The model under review builds one solid part; all positions refer to its coordinate system, in mm. Round coordinates to 2 decimals unless told otherwise and drop trailing zeros. Write each loop counter-clockwise with the first axis right and the second up, starting at its lowest first coordinate (ties: lowest second). Pieces come first, ordered by that corner, then holes. Notation, with made-up numbers: (58.25, -38.5) - (112.25, -38.5) arc R26 cw to (112.25, -17.5) - close; hole circle Ø10 at (46.5, 16). An arc over 180 degrees is marked (long way). Use one line per item in the form item = value.
from build123d import *

# Parameters (mm, degrees)
BOSS_EXTRUDE1_DEPTH = 5


with BuildPart() as part:
    # Sketch1 → Boss-Extrude1 (new body)
    with BuildSketch(Plane(origin=(0, 0, 0), x_dir=(1, 0, 0), z_dir=(0, 1, 0))):
        with BuildLine():
            ThreePointArc((-7.859375, 1.493393655), (-5.656854249, 5.656854249), (-1.493393655, 7.859375))
            ThreePointArc((-1.493393655, 7.859375), (-1.109264959, 9.009718401), (0, 9.5))
            Line((0, 9.5), (0, 15))
            ThreePointArc((0, 15), (-15, 0), (0, -15))
            Line((0, -15), (0, -9.5))
            ThreePointArc((0, -9.5), (-1.109264959, -9.009718401), (-1.493393655, -7.859375))
            ThreePointArc((-1.493393655, -7.859375), (-5.656854249, -5.656854249), (-7.859375, -1.493393655))
            ThreePointArc((-7.859375, -1.493393655), (-9.5, 0), (-7.859375, 1.493393655))
        make_face()
        with BuildLine():
            ThreePointArc((1.5, 8), (1.498347504, 7.929609954), (1.493393655, 7.859375))
            ThreePointArc((1.493393655, 7.859375), (5.656854249, 5.656854249), (7.859375, 1.493393655))
            ThreePointArc((7.859375, 1.493393655), (9.009718401, 1.109264959), (9.5, 0))
            ThreePointArc((9.5, 0), (9.009718401, -1.109264959), (7.859375, -1.493393655))
            ThreePointArc((7.859375, -1.493393655), (5.656854249, -5.656854249), (1.493393655, -7.859375))
            ThreePointArc((1.493393655, -7.859375), (1.498347504, -7.929609954), (1.5, -8))
            ThreePointArc((1.5, -8), (1.060660172, -9.060660172), (0, -9.5))
            Line((0, -9.5), (0, -15))
            ThreePointArc((0, -15), (10.606601718, -10.606601718), (15, 0))
            ThreePointArc((15, 0), (10.606601718, 10.606601718), (0, 15))
            Line((0, 15), (0, 9.5))
            ThreePointArc((0, 9.5), (1.060660172, 9.060660172), (1.5, 8))
        make_face()
        with BuildLine():
            ThreePointArc((0, -5), (-5, 0), (0, 5))
            Line((0, 5), (0, 6.5))
            ThreePointArc((0, 6.5), (-1.009718401, 6.890735041), (-1.493393655, 7.859375))
            ThreePointArc((-1.493393655, 7.859375), (-5.656854249, 5.656854249), (-7.859375, 1.493393655))
            ThreePointArc((-7.859375, 1.493393655), (-6.890735041, 1.009718401), (-6.5, 0))
            ThreePointArc((-6.5, 0), (-6.890735041, -1.009718401), (-7.859375, -1.493393655))
            ThreePointArc((-7.859375, -1.493393655), (-5.656854249, -5.656854249), (-1.493393655, -7.859375))
            ThreePointArc((-1.493393655, -7.859375), (-1.009718401, -6.890735041), (0, -6.5))
            Line((0, -6.5), (0, -5))
        make_face()
        with BuildLine():
            Line((0, 6.5), (0, 5))
            ThreePointArc((0, 5), (3.535533906, 3.535533906), (5, 0))
            ThreePointArc((5, 0), (3.535533906, -3.535533906), (0, -5))
            Line((0, -5), (0, -6.5))
            ThreePointArc((0, -6.5), (1.009718401, -6.890735041), (1.493393655, -7.859375))
            ThreePointArc((1.493393655, -7.859375), (5.656854249, -5.656854249), (7.859375, -1.493393655))
            ThreePointArc((7.859375, -1.493393655), (6.5, 0), (7.859375, 1.493393655))
            ThreePointArc((7.859375, 1.493393655), (5.656854249, 5.656854249), (1.493393655, 7.859375))
            ThreePointArc((1.493393655, 7.859375), (1.009718401, 6.890735041), (0, 6.5))
        make_face()
        with BuildLine():
            Line((40, 15), (0, 15))
            ThreePointArc((0, 15), (10.606601718, 10.606601718), (15, 0))
            ThreePointArc((15, 0), (10.606601718, -10.606601718), (0, -15))
            Line((0, -15), (40, -15))
            Line((40, -15), (40, 15))
        make_face()
    extrude(amount=BOSS_EXTRUDE1_DEPTH)


solid = part.part
(1) Add section C-C on z = 3.5. Write out the cut boundary in (x, y).
Geometry results:
outline = (-14.59, 0) - (-3.57, 0) - (-3.57, 5) - (-14.59, 5) - close; (3.57, 0) - (40, 0) - (40, 5) - (3.57, 5) - close
(2) Add section A-A on y = 4.1. Write out the cut boundary in (x, z).
Geometry results:
outline = (0, -15) - (40, -15) - (40, 15) - (0, 15) arc R15 ccw to start; hole circle Ø3 at (-8, 0); hole circle Ø10 at (0, 0); hole circle Ø3 at (0, -8); hole circle Ø3 at (0, 8); hole circle Ø3 at (8, 0)
(3) To check wall thickness, follow L1, parallel to X at y = 3.6, z = -1.25; L2, parallel to Z at x = -8, y = 2; L3, parallel to X at y = 4.3, z = -1.75. State the ranges of each line that lie inside material, in increasing order.
Geometry results:
L1 = -14.95 to -8.83, -7.17 to -4.84, 4.84 to 7.17, 8.83 to 40
L2 = -12.69 to -1.5, 1.5 to 12.69
L3 = -14.9 to -4.68, 4.68 to 40
(4) Insertion check: P1, Ø2.5, axis at x = -8, z = 0, coming from the +Y side; P2, Ø2, axis at y = 3, z = -3, coming from the -X side. Each pin has a flat end and moves straight along its axis. Give the tip position at first contact, or say it passes through.
Geometry results:
P1 = through
P2 = -14.87
(5) Add section B-B on z = -4.25. Write out the cut boundary in (x, y).
Geometry results:
outline = (-14.39, 0) - (-2.63, 0) - (-2.63, 5) - (-14.39, 5) - close; (2.63, 0) - (40, 0) - (40, 5) - (2.63, 5) - close
(6) Add section D-D on x = -10.5. Write out the cut boundary in (y, z), then the cut area to 3 significant figures.
Geometry results:
outline = (0, -10.71) - (5, -10.71) - (5, 10.71) - (0, 10.71) - close
area = 107 mm2
